Work out the finished part from the listing and answer in its coordinate system (mm). Face numbers are marked on the shaded views. A direction names the side the tool comes from. Give positions to 0.01 mm unless a question says otherwise; leave off trailing zeros. Order: outer loops, then holes, each group sorted by start corner. A loop starts at its lowest first (then second) coordinate and runs counter-clockwise, first axis right, second up. Notation, with made-up numbers: (50.25, 63) - (84.25, 63) arc R26 cw to (84.25, 96) - close; hole circle Ø9 at (-15, 34.5). An arc over 180 degrees is marked (long way). Return JSON: item names as keys, results as strings. Group by question number.
Autodesk Inventor part; units mm, degrees
ref_plane "YZ Plane" through (0, 0, 0) normal (1, 0, 0) x (0, 1, 0)
ref_plane "XZ Plane" through (0, 0, 0) normal (0, 1, 0) x (-1, 0, 0)
ref_plane "XY Plane" through (0, 0, 0) normal (0, 0, 1) x (1, 0, 0)
sketch "Sketch1" plane through (0, 0, 0) normal (0, 1, 0) x (-1, 0, 0)
  line L0 (-6, 20) -> (-6, 0)
  line L1 (-6, 0) -> (14, -6)
  line L2 (14, -6) -> (14, -53)
  line L3 (14, -53) -> (10, -53)
  line L4 (10, -53) -> (10, -10)
  line L5 (-10, -10) -> (-10, 20)
  line L6 (-10, 20) -> (-6, 20)
  line L7 (10, -10) -> (-10, -10)
  point P0 (0, 0)
  point P1 (0, -10)
  dimension "d0" = 20
  dimension "d1" = 43
  dimension "d2" = 4
  dimension "d3" = 4
  dimension "d4" = 30
  dimension "d5" = 20
  dimension "d6" = 4
extrude "Extrusion1" add sketch "Sketch1" along normal mid plane 44
sketch "Sketch2" plane through (-14, -22, -6) normal (-1, 0, 0) x (0, 0, 1)
  line L0 (0, 44) -> (0, 0)
  line L1 (-47, 44) -> (0, 44)
  line L2 (-47, 44) -> (-47, 0)
  line L3 (0, 0) -> (-47, 0)
  circle A0 centre (-25.85, 22) radius 12.5
  circle A1 centre (-41.35, 37.5) radius 1.6
  circle A2 centre (-41.35, 6.5) radius 1.6
  circle A3 centre (-10.35, 37.5) radius 1.6
  circle A4 centre (-10.35, 6.5) radius 1.6
  point P0 (6, 22)
  point P1 (-47, 22)
  dimension "d9" = 3.2
  dimension "d10" = 25
  dimension "d11" = 21.15
  dimension "d12" = 31
  dimension "d13" = 31
  dimension "d14" = 15.5
  dimension "d15" = 15.5
extrude "Extrusion2" cut sketch "Sketch2" against normal up to next contours A0 | A1 | A2 | A3 | A4
sketch "Sketch3" plane through (6, -22, 20) normal (-1, 0, 0) x (0, 0, 1)
  arc A0 (-5.7957, 34.4085) -> (-5.6306, 37.6) centre (-5.6306, 36) ccw
  arc A1 (-9.6306, 37.6) -> (-9.7957, 34.4085) centre (-9.7957, 36.0085) ccw
  arc A2 (-5.6306, 20.4) -> (-5.6306, 23.6) centre (-5.6306, 22) ccw
  arc A3 (-9.7957, 23.6) -> (-9.7957, 20.4) centre (-9.7957, 22) ccw
  arc A4 (-5.6306, 6.4) -> (-5.6306, 9.6) centre (-5.6306, 8) ccw
  arc A5 (-9.7957, 9.6) -> (-9.7957, 6.4) centre (-9.7957, 8) ccw
  line L0 (-9.6306, 37.6) -> (-5.6306, 37.6)
  line L1 (-9.7957, 34.4085) -> (-5.7957, 34.4085)
  line L2 (-9.7957, 23.6) -> (-5.6306, 23.6)
  line L3 (-9.7957, 20.4) -> (-5.6306, 20.4)
  line L4 (-9.7957, 9.6) -> (-5.6306, 9.6)
  line L5 (-9.7957, 6.4) -> (-5.6306, 6.4)
  line L6 (-20, 44) -> (0, 44)
  line L7 (0, 0) -> (-20, 0)
  line L8 (-5.6306, 36) -> (-5.6306, 8) construction
  point P0 (-20, 22)
  dimension "d18" = 3.2
  dimension "d19" = 4
  dimension "d20" = 8
  dimension "d21" = 8
extrude "Extrusion3" cut sketch "Sketch3" against normal up to next
sketch "Sketch4" plane through (-14, -22, -6) normal (-1, 0, 0) x (0, 0, 1)
  line L0 (0, 44) -> (0, 0)
  line L1 (0, 40) -> (8.5563, 40)
  line L2 (8.5563, 40) -> (8.5563, 4)
  line L3 (8.5563, 4) -> (0, 4)
  line L4 (0, 4) -> (0, 40)
  point P0 (6, 22)
  dimension "d26" = 4
  dimension "d27" = 4
extrude "Extrusion4" cut sketch "Sketch4" against normal up to surface (20 mm away)
fillet "Fillet1" radius 2 4 edges at (-12, 22, -53) (-12, -22, -53) (8, -22, 20) (8, 22, 20)
equation "\"d14\" = 0.5 * d13"
equation "\"d15\" = 0.5 * d12"
properties part number "nema17-mount-bottom-z-axis"
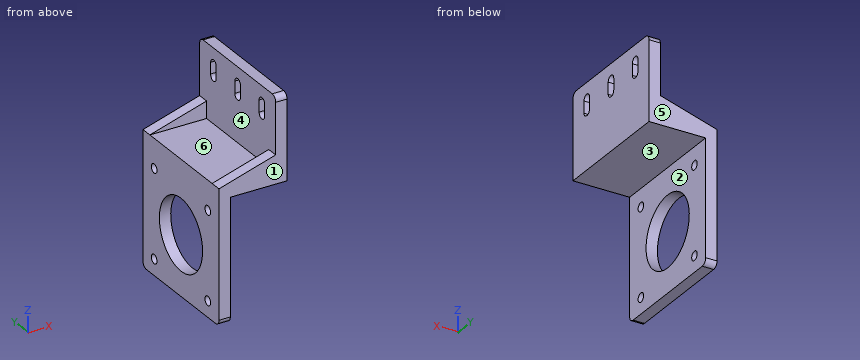
1. Consider probe 1 along Y at (x, z) = (-11.7, -16.35); probe 2 along Y at (x, z) = (-9.75, -5.5); probe 3 along Y at (x, z) = (-13, -31.85). Determine where each line is inside the solid, lowest interval first. Write a range as from..to.
2. A tool of negligible diameter and unlimited length cuts with its end or side. For the marked faces 1 and 2, from which of +Z, -Z, +X, -X, +Y, -Y can it reach the whole face along a straight path? Write none if from no direction.
3. The part is cut by section C-C (z = -16.35). Give the vertices of the cut face in (x, y).
4. The part is cut by section A-A (y = 0). Give the vertices of the cut face in (x, z), and give its area (3 significant figures).
5. Determine the mould class of the marked faces 3, 4, 5 and 6 for opening direction Y: released by +Y, released by -Y, zero draft, split by the parting line, or undercut.
6. The part is cut by section B-B (x = -12.5). Give the vertices of the cut face in (y, z), and give its area (3 significant figures).
7. The part is cut by section D-D (z = -33.5). Give the vertices of the cut face in (x, y).
8. Each of these flat-tipped pins is pushed along its axis until it touches: pin 1 (10 mm diameter, centred on x = 1.5, y = 5, fed in from -Z); pin 2 (6 mm diameter, centred on x = 0.5, y = 9, fed in from +Z); pin 3 (8 mm diameter, centred on y = 7.5, z = 8, fed in from -X). Where does it stop, or does it pass through?
Answers:
{
 "1": {"probe 1": "y = -22..-17.1, -13.9..13.9, 17.1..22", "probe 2": "y = -22..-18, 18..22", "probe 3": "y = -22..-12.5, 12.5..22"},
 "2": {"face 1": "+Z, -Z, +X, -X, -Y", "face 2": "-Z, +X, +Y, -Y"},
 "3": {"outline": "(-14, -22) - (-10, -22) - (-10, -17.1) - (-14, -17.1) - close; (-14, -13.9) - (-10, -13.9) - (-10, 13.9) - (-14, 13.9) - close; (-14, 17.1) - (-10, 17.1) - (-10, 22) - (-14, 22) - close"},
 "4": {"outline": "(-14, -53) - (-10, -53) - (-10, -44.35) - (-14, -44.35) - close; (-14, -19.35) - (-10, -19.35) - (-10, -10) - (10, -10) - (10, 8.6) - (6, 8.6) - (6, -6) - (-14, -6) - close; (6, 15.97) - (10, 15.97) - (10, 20) - (6, 20) - close", "area": "243 mm^2"},
 "5": {"face 3": "zero draft", "face 4": "undercut", "face 5": "released by +Y", "face 6": "undercut"},
 "6": {"outline": "(-22, -51) arc R2 ccw to (-20, -53) - (20, -53) arc R2 ccw to (22, -51) - (22, -5.55) - (18, -5.55) - (18, -6) - (-18, -6) - (-18, -5.55) - (-22, -5.55) - close; hole circle Ø3.2 at (-15.5, -47.35); hole circle Ø3.2 at (-15.5, -16.35); hole circle Ø25 at (0, -31.85); hole circle Ø3.2 at (15.5, -47.35); hole circle Ø3.2 at (15.5, -16.35)", "area": "1,550 mm^2"},
 "7": {"outline": "(-14, -22) - (-10, -22) - (-10, -12.39) - (-14, -12.39) - close; (-14, 12.39) - (-10, 12.39) - (-10, 22) - (-14, 22) - close"},
 "8": {"pin 1": "stops at z = -10", "pin 2": "stops at z = -6", "pin 3": "stops at x = 6"}
}
